Read the model definition and answer for the solid it produces. Units are mm, in the model's axes. A direction names the side the tool comes from. Coordinates: 2 decimals unless noted, no trailing zeros. Write each loop counter-clockwise with the first axis right and the second up, starting at its lowest first coordinate (ties: lowest second). Pieces come first, ordered by that corner, then holes.
Item 1: Section C-C (z = 1.5) is taken. Give the vertices of the cut face in (x, y), then the cut area to 3 significant figures.
Item 2: Section D-D (z = -0.5) is taken. Give the vertices of the cut face in (x, y), then the cut area to 3 significant figures.
Item 3: Straight lines are drawn through the part: probe 1 along X at (y, z) = (0.6, 0); probe 2 along X at (y, z) = (-4.5, -2.25); probe 3 along X at (y, z) = (0.85, 0). For each, find the intervals that lie inside material, in ascending order.
Item 4: Section B-B (y = -3.25) is taken. Give the vertices of the cut face in (x, z), then the cut area to 3 significant figures.
Item 5: Determine the mould class of faces 5 (the face through (-12, -2, -2)), 6 (the face through (22, 0, 0)), 7 (the face through (16, -2, 0)) for opening direction X: released by +X, released by -X, zero draft, split by the parting line, or undercut.
Item 6: Each of these flat-tipped pins is pushed along its axis until it touches: P1, Ø3, axis at x = 25.75, z = 0, coming from the -Y side; P2, Ø2.5, axis at y = -3.5, z = -0.5, coming from the +X side; P3, Ø2.5, axis at x = -16, y = -2, coming from the +Z side. Where does it stop, or does it pass through?
Item 7: A tool of negligible diameter and unlimited length cuts with its end or side. For faces 1 (the face through (3, -2, 0)), 2 (the face through (-15, -2, 0)), 3 (the face through (-27.715, 0.254, -3.699)), 4 (the face through (-18, -2, -2)), from which of +Z, -Z, +X, -X, +Y, -Y can it reach the whole face along a straight path? Write none if from no direction.
Item 8: Section A-A (x = 25.75) is taken. Give the vertices of the cut face in (y, z), then the cut area to 3 significant figures.
from build123d import *

# Parameters (mm, degrees)
SKETCH1_W               = 56
SKETCH1_H               = 8
BOSS_EXTRUDE1_DEPTH     = 1.5
CUT_EXTRUDE1_DEPTH      = 29.324018077
CUT_EXTRUDE1_DEPTH_BACK = 29.324018077
SKETCH2_R               = 1
FILLET1_R               = 1
SKETCH3_W               = 13
SKETCH3_H               = 8
SKETCH3_W_2             = 6
SKETCH3_H_2             = 4
BOSS_EXTRUDE2_DEPTH     = 5


with BuildPart() as part:
    # Sketch1 → Boss-Extrude1 (new body)
    with BuildSketch(Plane(origin=(0, 0, 0), x_dir=(1, 0, 0), z_dir=(0, 1, 0))):
        Rectangle(SKETCH1_W, SKETCH1_H)
    extrude(amount=BOSS_EXTRUDE1_DEPTH)

    # Sketch2 → Cut-Extrude1 (cut, two sides: drawn at the far end of the back side and taken through both)
    with BuildSketch(Plane(origin=(0, 1.5, 0), x_dir=(1, 0, 0), z_dir=(0, 1, 0)).offset(-CUT_EXTRUDE1_DEPTH_BACK)):
        with Locations(Location((-25.75, 0, 0), (0, 0, 270))):
            Circle(SKETCH2_R)
        with Locations(Location((25.75, 0, 0), (0, 0, 270))):
            Circle(SKETCH2_R)
    extrude(amount=CUT_EXTRUDE1_DEPTH + CUT_EXTRUDE1_DEPTH_BACK, mode=Mode.SUBTRACT)

    # Fillet1
    fillet1_edges = [part.edges().sort_by_distance(p)[0] for p in [
        (28, 1.5, 0),
        (0, 1.5, -4),
        (-28, 1.5, 0),
        (-28, 0.75, -4),
        (28, 0.75, -4),
        (28, 0.75, 4),
        (-28, 0.75, 4),
        (0, 1.5, 4),
    ]]
    fillet(fillet1_edges, radius=FILLET1_R)

    # Sketch3 → Boss-Extrude2 (add)
    with BuildSketch(Plane.XZ):
        with Locations((9.5, 0)):
            Rectangle(SKETCH3_W, SKETCH3_H)
        with Locations((-15, -2)):
            Rectangle(SKETCH3_W_2, SKETCH3_H_2)
    extrude(amount=BOSS_EXTRUDE2_DEPTH)


solid = part.part
Established:
1. outline: (-28, 0) - (3, 0) - (3, -5) - (16, -5) - (16, 0) - (28, 0) - (28, 0.5) arc R1 ccw to (27, 1.5) - (-27, 1.5) arc R1 ccw to (-28, 0.5) - close
1. area: 149 mm2
2. outline: (-28, 0) - (-26.62, 0) - (-26.62, 1.5) - (-27, 1.5) arc R1 ccw to (-28, 0.5) - close; (-24.88, 0) - (-18, 0) - (-18, -5) - (-12, -5) - (-12, 0) - (3, 0) - (3, -5) - (16, -5) - (16, 0) - (24.88, 0) - (24.88, 1.5) - (-24.88, 1.5) - close; (26.62, 0) - (28, 0) - (28, 0.5) arc R1 ccw to (27, 1.5) - (26.62, 1.5) - close
2. area: 173 mm2
3. probe 1: x = -27.99 to -26.75, -24.75 to 24.75, 26.75 to 27.99
3. probe 2: x = -18 to -12, 3 to 16
3. probe 3: x = -27.94 to -26.75, -24.75 to 24.75, 26.75 to 27.94
4. outline: (-18, -4) - (-12, -4) - (-12, 0) - (-18, 0) - close; (3, -4) - (16, -4) - (16, 4) - (3, 4) - close
4. area: 128 mm2
5. face 5: undercut
5. face 6: zero draft
5. face 7: released by +X
6. P1: stops at y = 0
6. P2: stops at x = 16
6. P3: stops at z = 0
7. face 1: +Z, -Z, -Y
7. face 2: +Z, -X, -Y
7. face 3: -Z, -X, +Y, -Y
7. face 4: +Z, -Z, -X, -Y
8. outline: (0, -4) - (0.5, -4) arc R1 ccw to (1.5, -3) - (1.5, -1) - (0, -1) - close; (0, 1) - (1.5, 1) - (1.5, 3) arc R1 ccw to (0.5, 4) - (0, 4) - close
8. area: 8.57 mm2
